Can you work these out from the model? Positions are in its coordinate system, mm. Give positions to 0.01 mm unless a question says otherwise; leave off trailing zeros. Loops run counter-clockwise (first coordinate to the right, second up) from the corner with the lowest first, then second, coordinate; pieces in that order, holes last. Notation, with made-up numbers: M 47,-29.5 L 103,-29.5 A14 cw 103,-12.5 Z; hole C 55.5,-39 d8. An arc over 180 degrees is marked long. Use CSV: the item, a comma, the result in double quotes.
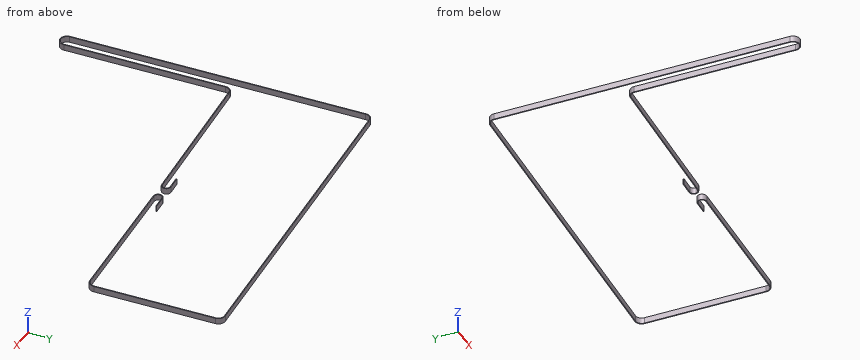
Autodesk Inventor part; units mm, degrees
ref_plane "Work Plane2" through (204.3918, -104.9631, 0) normal (0.9984426, 0.0557893, 0) x (-0.0557893, 0.9984426, 0)
ref_plane "YZ Plane" through (0, 0, 0) normal (1, 0, 0) x (0, 1, 0)
ref_plane "XZ Plane" through (0, 0, 0) normal (0, 1, 0) x (-1, 0, 0)
sketch "Sketch1" plane through (0, 0, 0) normal (0, 0, 1) x (1, 0, 0)
  circle A0 centre (0, 0) radius 6.05
surface extrude "ExtrusionSrf1" sketch "Sketch1" along normal mid plane 6 shown yes curves A0
sketch "Sketch2" plane through (0, 0, 0) normal (0, 0, 1) x (1, 0, 0)
  circle A0 centre (324.3803, 20.0598) radius 6.05
  point P0 (0, 0)
surface extrude "ExtrusionSrf2" sketch "Sketch2" along normal mid plane 6 shown yes curves A0
sketch "Sketch3" plane through (0, 0, 0) normal (0, 0, 1) x (1, 0, 0)
  circle A0 centre (18.0229, -291.4433) radius 6.11
  point P0 (0, 0)
surface extrude "ExtrusionSrf3" sketch "Sketch3" along normal blind 6 shown yes curves A0
sketch "Sketch4" plane through (0, 0, 0) normal (0, 0, 1) x (1, 0, 0)
  circle A0 centre (20.8883, -131.5327) radius 5.735
  point P0 (0, 0)
surface extrude "ExtrusionSrf4" sketch "Sketch4" along normal mid plane 6 shown yes curves A0
sketch "Sketch5" plane through (0, 0, 0) normal (0, 0, 1) x (1, 0, 0)
  circle A0 centre (331.7772, -99.5529) radius 6.05
  point P0 (0, 0)
surface extrude "ExtrusionSrf5" sketch "Sketch5" along normal mid plane 6 shown yes curves A0
sketch "Sketch6" plane through (0, 0, 0) normal (0, 0, 1) x (1, 0, 0)
  circle A0 centre (172.6717, -110.8599) radius 3
  point P0 (0, 0)
surface extrude "ExtrusionSrf6" sketch "Sketch6" along normal mid plane 6 shown yes curves A0
sketch "Sketch7" plane through (0, 0, 0) normal (0, 0, 1) x (1, 0, 0)
  circle A0 centre (191.6355, -109.6871) radius 3
  point P0 (0, 0)
surface extrude "ExtrusionSrf7" sketch "Sketch7" along normal mid plane 6 shown yes curves A0
sketch "Sketch8" plane through (0, 0, 0) normal (0, 0, 1) x (1, 0, 0)
  circle A0 centre (0, 0) radius 6.05
  circle A1 centre (20.8883, -131.5327) radius 5.735
  circle A2 centre (18.0229, -291.4433) radius 6.11
  circle A3 centre (172.6717, -110.8599) radius 3
  circle A4 centre (191.6355, -109.6871) radius 3
  circle A5 centre (331.7772, -99.5529) radius 6.05
  circle A6 centre (324.3803, 20.0598) radius 6.05
  arc A7 (-0.3892, 6.293) -> (-6.2931, -0.3879) centre (0, 0) ccw
  arc A8 (11.67, -291.8348) -> (24.3758, -291.0504) centre (18.0229, -291.4433) ccw
  arc A9 (20.4583, -125.1822) -> (14.5355, -131.9256) centre (20.8883, -131.5327) ccw
  arc A10 (172.9424, -114.8557) -> (172.4011, -106.864) centre (172.6717, -110.8599) ccw
  arc A11 (330.6733, 20.4489) -> (323.9912, 26.3527) centre (324.3803, 20.0598) ccw
  arc A12 (191.4121, -105.6884) -> (191.859, -113.6859) centre (191.6355, -109.6871) ccw
  arc A13 (332.129, -105.8481) -> (338.0702, -99.1638) centre (331.7772, -99.5529) ccw
  line L0 (11.67, -291.8348) -> (-6.2931, -0.3879)
  line L1 (-0.3892, 6.293) -> (323.9912, 26.3527)
  line L2 (24.3758, -291.0504) -> (14.5355, -131.9256)
  line L3 (20.4583, -125.1822) -> (172.9424, -114.8557)
  line L4 (330.6733, 20.4489) -> (338.0702, -99.1638)
  line L5 (159.4309, -107.7424) -> (172.4011, -106.864)
  line L6 (191.859, -113.6859) -> (332.129, -105.8481)
  line L7 (191.4121, -105.6884) -> (204.3918, -104.9631)
  dimension "d14" = 0.255
  dimension "d15" = 0.255
  dimension "d16" = 0.255
  dimension "d17" = 0.63
  dimension "d19" = 0.255
  dimension "d22" = 1.005
  dimension "d23" = 1.005
  dimension "d34" = 13
  dimension "d35" = 13
ref_plane "Work Plane2" through (204.3918, -104.9631, 0) normal (0.9984426, 0.0557893, 0) x (-0.0557893, 0.9984426, 0)
sketch "Sketch10" plane through (204.3918, -104.9631, 0) normal (0.9984426, 0.0557893, 0) x (-0.0557893, 0.9984426, 0)
  line L0 (0.63, 3) -> (-0.255, 3)
  line L1 (-0.255, 3) -> (-0.255, -3)
  line L2 (-0.255, -3) -> (0.63, -3)
  line L3 (0.63, -3) -> (0.63, 3)
  line L4 (0.63, 0) -> (-0.255, 0) construction
  point P0 (116.2025, 0)
  point P1 (0, 0)
  dimension "d29" = 6
  dimension "d30" = 0.63
  dimension "d31" = 0.255
sweep "Sweep2" add profiles "Sketch10" path "Sketch8" path curves L7 A12 L6 A13 L4 A11 L1 A7 L0 A8 L2 A9 L3 A10 L5
equation "\"d14\" = inside"
equation "\"d15\" = inside"
equation "\"d16\" = inside"
equation "\"d17\" = backside"
equation "\"d19\" = inside"
equation "\"inside\" = 0.255"
equation "\"backside\" = 0.63"
properties part number "Belt 4" material "Rubber"
Q1. I'm going to push flat-ended pins straight in: P1, Ø3, axis at y = -14, z = 1.5, coming from the +X side; P2, Ø1, axis at y = -183.5, z = -2, coming from the -X side; P3, Ø1, axis at x = 71.5, z = -1, coming from the +Y side. Where does each tip first touch, or does it pass through?
Model answer:
P1,"x = 333.53"
P2,"x = 4.33"
P3,"y = 11.4"
Q2. I want a section at C-C, the plane y = -42. Please give me the cut outline in (x, z), then the cut area to 3 significant figures.
Model answer:
outline,"M -4.36,-3 L -3.47,-3 L -3.47,3 L -4.36,3 Z; M 334.28,-3 L 335.17,-3 L 335.17,3 L 334.28,3 Z"
area,"10.6 mm2"
Q3. I want a section at A-A, the plane x = 297. Please give me the cut outline in (y, z).
Model answer:
outline,"M -108.44,-3 L -107.56,-3 L -107.56,3 L -108.44,3 Z; M 24.43,-3 L 25.31,-3 L 25.31,3 L 24.43,3 Z"
Q4. Please list where these lines run through material, in increasing order: L1, parallel to Y at x = 166.5, z = 2.5; L2, parallel to X at y = -147.5, z = 0.05; L3, parallel to Y at x = 126.5, z = 1.9. Write a range as from..to.
Model answer:
L1,"-115.92..-115.04, -107.52..-106.63, 16.36..17.24"
L2,"2.14..3.03, 15.24..16.13"
L3,"-118.63..-117.75, 13.88..14.77"
